Geometry check sheet. Reference: the model listing, model coordinates, mm. Face numbers are marked on the shaded views. A direction names the side the tool comes from. Coordinates: 2 decimals unless noted, no trailing zeros. Loops run counter-clockwise (first coordinate to the right, second up) from the corner with the lowest first, then second, coordinate; pieces in that order, holes last.
from build123d import *
from build123d.topology import SkipClean

# Parameters (mm, degrees)
BOSS_EXTRUDE1_DEPTH      = 42.5
BOSS_EXTRUDE1_DEPTH_BACK = 15
SKETCH1_W                = 40
SKETCH1_H                = 65
SKETCH3_W                = 22.5
SKETCH3_H                = 50
CUT_EXTRUDE2_DEPTH       = 30
SKETCH4_R                = 4.5
CUT_EXTRUDE3_DEPTH       = 10
SKETCH5_W                = 35
SKETCH5_H                = 25
BOSS_EXTRUDE3_DEPTH      = 15
SKETCH6_R                = 3
CUT_EXTRUDE4_DEPTH       = 30
CUT_EXTRUDE5_DEPTH       = 108.964114408
BOSS_EXTRUDE4_DEPTH      = 10
BOSS_EXTRUDE5_OUTLINE_R  = 3
BOSS_EXTRUDE5_DEPTH      = 50
BOSS_EXTRUDE6_START      = -35
SKETCH11_R               = 3
BOSS_EXTRUDE6_DEPTH      = 35
SKETCH12_W               = 14
SKETCH12_H               = 65
SKETCH12_R               = 3.1
SKETCH12_W_2             = 75
SKETCH12_H_2             = 14
BOSS_EXTRUDE7_DEPTH      = 5
SKETCH13_R               = 1.6
CUT_EXTRUDE6_DEPTH       = 115.988042857
CUT_EXTRUDE7_DEPTH       = 12.25
CUT_EXTRUDE7_DEPTH_BACK  = 12.25
SKETCH14_W               = 43.75
SKETCH14_H               = 50
CUT_EXTRUDE8_DEPTH       = 30
CUT_EXTRUDE9_DEPTH       = 115.988042857


# Read off the part's stored shape, not the designer's step: Boss-Extrude5
with BuildPart() as part:
    # Sketch1 → Boss-Extrude1 (new, two sides: drawn at the far end of the back side and taken through both)
    with BuildSketch(Plane.XY.offset(-BOSS_EXTRUDE1_DEPTH_BACK)):
        with Locations((20, 32.5)):
            Rectangle(SKETCH1_W, SKETCH1_H)
    extrude(amount=BOSS_EXTRUDE1_DEPTH + BOSS_EXTRUDE1_DEPTH_BACK)

    # Sketch3 → Cut-Extrude2 (cut)
    with BuildSketch(Plane(origin=(40, 0, 0), x_dir=(0, 0, -1), z_dir=(1, 0, 0))):
        with Locations((-11.25, 40)):
            Rectangle(SKETCH3_W, SKETCH3_H)
    extrude(amount=-CUT_EXTRUDE2_DEPTH, mode=Mode.SUBTRACT)

    # Sketch4 → Cut-Extrude3 (cut)
    with BuildSketch(Plane(origin=(10, 0, 0), x_dir=(0, 0, -1), z_dir=(1, 0, 0))):
        with Locations((-11.25, 26.5)):
            Circle(SKETCH4_R)
    extrude(amount=-CUT_EXTRUDE3_DEPTH, mode=Mode.SUBTRACT)

    # Sketch5 → Boss-Extrude3 (add)
    with BuildSketch(Plane.XZ):
        with Locations((57.5, 30)):
            Rectangle(SKETCH5_W, SKETCH5_H)
    extrude(amount=-BOSS_EXTRUDE3_DEPTH)

    # Sketch6 → Cut-Extrude4 (cut)
    with BuildSketch(Plane.XZ):
        with Locations(Location((32, 29.5, 0), (0, 0, 270))):
            Circle(SKETCH6_R)
        with Locations(Location((64, 29.5, 0), (0, 0, 270))):
            Circle(SKETCH6_R)
    extrude(amount=-CUT_EXTRUDE4_DEPTH, mode=Mode.SUBTRACT)

    # Sketch8 → Cut-Extrude5 (cut, through all)
    with BuildSketch(Plane.XZ):
        Polygon((48.25, 17.5), (42.75, 17.5), (42.75, 23), (53.75, 23), (53.75, 17.5), align=None)
    extrude(amount=-CUT_EXTRUDE5_DEPTH, mode=Mode.SUBTRACT)

    # Sketch9 → Boss-Extrude4 (add)
    with BuildSketch(Plane.XY.offset(42.5)):
        Polygon((0, 65), (0, 0), (75, 0), (75, 15), (40, 15), (40, 65), align=None)
    extrude(amount=BOSS_EXTRUDE4_DEPTH)

    # Boss-Extrude5 outline → Boss-Extrude5 (add)
    with SkipClean():  # the faces are left unmerged after this step: merging them gives an invalid solid
        with BuildSketch(Plane(origin=(0, 15, 0), x_dir=(1, 0, 0), z_dir=(0, 1, 0))):
            Polygon((75, -52.5), (75, -22.5), (53.75, -22.5), (53.75, -23), (42.75, -23), (42.75, -22.5), (40, -22.5), (40, -52.5), align=None)
            with Locations((64, -29.5)):
                Circle(BOSS_EXTRUDE5_OUTLINE_R, mode=Mode.SUBTRACT)
        extrude(amount=BOSS_EXTRUDE5_DEPTH)

    # Sketch11 → Boss-Extrude6 (add)
    with SkipClean():  # the faces are left unmerged after this step: merging them gives an invalid solid
        with BuildSketch(Plane(origin=(0, 65, 0), x_dir=(1, 0, 0), z_dir=(0, 1, 0)).offset(BOSS_EXTRUDE6_START)):
            with Locations(Location((64, -29.5, 0), (0, 0, 90))):
                Circle(SKETCH11_R)
        extrude(amount=BOSS_EXTRUDE6_DEPTH)

    # Sketch12 → Boss-Extrude7 (add)
    # profile 1 of 2: a face of its own
    with SkipClean():  # the faces are left unmerged after this step: merging them gives an invalid solid
        with BuildSketch(Plane.XY.offset(52.5)):
            with Locations((82, 32.5)):
                Rectangle(SKETCH12_W, SKETCH12_H)
            with Locations((82, 53)):
                Circle(SKETCH12_R, mode=Mode.SUBTRACT)
            with Locations((82, 12)):
                Circle(SKETCH12_R, mode=Mode.SUBTRACT)
        # profile 2 of 2: a face of its own
        with BuildSketch(Plane.XY.offset(52.5)):
            with Locations((37.5, -7)):
                Rectangle(SKETCH12_W_2, SKETCH12_H_2)
            with Locations((12, -7)):
                Circle(SKETCH12_R, mode=Mode.SUBTRACT)
            with Locations((63, -7)):
                Circle(SKETCH12_R, mode=Mode.SUBTRACT)
        extrude(amount=-BOSS_EXTRUDE7_DEPTH)

    # Sketch13 → Cut-Extrude6 (cut, through all)
    with SkipClean():  # the faces are left unmerged after this step: merging them gives an invalid solid
        with BuildSketch(Plane(origin=(10, 0, 0), x_dir=(0, 0, -1), z_dir=(1, 0, 0))):
            with Locations((-2.5, 47)):
                Circle(SKETCH13_R)
            with Locations((-20, 47)):
                Circle(SKETCH13_R)
        extrude(amount=-CUT_EXTRUDE6_DEPTH, mode=Mode.SUBTRACT)

    # Sketch14 → Cut-Extrude7 (cut, two sides: drawn at the far end of the back side and taken through both)
    with SkipClean():  # the faces are left unmerged after this step: merging them gives an invalid solid
        with BuildSketch(Plane(origin=(0, 0, 11.25), x_dir=(-1, 0, 0), z_dir=(0, 0, -1)).offset(-CUT_EXTRUDE7_DEPTH_BACK)):
            with Locations((-31.875, 40)):
                Rectangle(SKETCH14_W, SKETCH14_H)
        extrude(amount=CUT_EXTRUDE7_DEPTH + CUT_EXTRUDE7_DEPTH_BACK, mode=Mode.SUBTRACT)

    # Sketch15 → Cut-Extrude8 (cut)
    with SkipClean():  # the faces are left unmerged after this step: merging them gives an invalid solid
        with BuildSketch(Plane(origin=(40, 0, 0), x_dir=(0, 0, -1), z_dir=(1, 0, 0))):
            Polygon((-11.25, 15), (-8.25, 15), (-8.25, 9), (-14.25, 9), (-14.25, 15), align=None)
        extrude(amount=-CUT_EXTRUDE8_DEPTH, mode=Mode.SUBTRACT)

    # Sketch16 → Cut-Extrude9 (cut, through all)
    with SkipClean():  # the faces are left unmerged after this step: merging them gives an invalid solid
        with BuildSketch(Plane(origin=(10, 0, 0), x_dir=(0, 0, -1), z_dir=(1, 0, 0))):
            Polygon((-11.25, 65), (-8.25, 65), (-8.25, 50), (-14.25, 50), (-14.25, 65), align=None)
        extrude(amount=-CUT_EXTRUDE9_DEPTH, mode=Mode.SUBTRACT)


solid = part.part
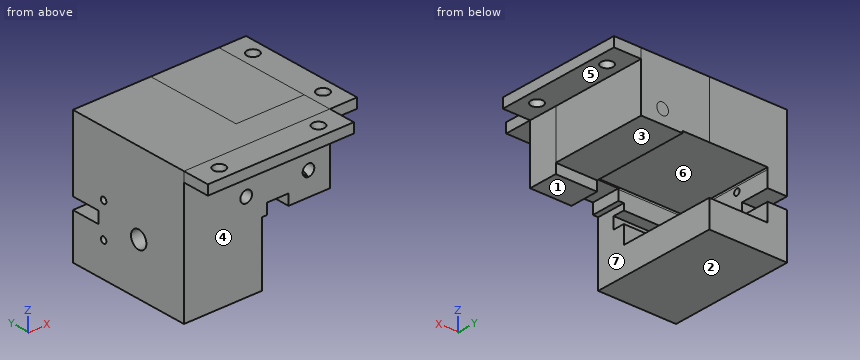
(1) Access from +Z, -Z, +X, -X, +Y, -Y to the whole of each face (thin tool, end or side, straight path). Record for the marked faces 1, 2, 3 and 4.
Findings:
face 1: -Z, +X, +Y, -Y
face 2: -Z, +X, -X, +Y, -Y
face 3: -Z, +X, +Y
face 4: -Z, +X, -X, -Y
(2) Sectioned sample at C-C on x = 12. Record the cut outline in (y, z), and give its area (3 significant figures).
Findings:
outline: (-14, 47.5) - (-10.1, 47.5) - (-10.1, 52.5) - (-14, 52.5) - close; (-3.9, 47.5) - (0, 47.5) - (0, -15) - (65, -15) - (65, -1) - (15, -1) - (15, 8.25) - (9, 8.25) - (9, 14.25) - (15, 14.25) - (15, 23.5) - (65, 23.5) - (65, 52.5) - (-3.9, 52.5) - close
area: 3,170 mm2
(3) Sectioned sample at D-D on z = 20. Record the cut outline in (x, y).
Findings:
outline: (0, 0) - (42.75, 0) - (42.75, 15) - (10, 15) - (10, 45.4) - (0, 45.4) - close; (0, 48.6) - (10, 48.6) - (10, 65) - (0, 65) - close; (53.75, 0) - (75, 0) - (75, 15) - (53.75, 15) - close
(4) Gauge pin test, flat ends, axial feed: pin 1 Ø8 at (x, z) = (34, 16.5) entering from -Y; pin 2 Ø3 at (x, z) = (30, 6.5) entering from +Y; pin 3 Ø12.5 at (y, z) = (48, 38.5) entering from +X; pin 4 Ø11.5 at (y, z) = (26.5, 11.25) entering from -X. Record the tip position at first contact, or that the pin passes through.
Findings:
pin 1: stops at y = 0
pin 2: stops at y = 15
pin 3: stops at x = 75
pin 4: stops at x = 0
(5) Draft check along X on the marked faces 5, 6 and 7. Enter one of: +X half, -X half, draft (parallel to the pull), parting line (faces both ways), or undercut.
Findings:
face 5: draft
face 6: undercut
face 7: +X half
(6) Sectioned sample at B-B on z = 11.25. Record the cut outline in (x, y), and give its area (3 significant figures).
Findings:
outline: (0, 0) - (40, 0) - (40, 9) - (10, 9) - (10, 22) - (0, 22) - close; (0, 31) - (10, 31) - (10, 50) - (0, 50) - close
area: 680 mm2
(7) Sectioned sample at A-A on y = 26.5. Record the cut outline in (x, z).
Findings:
outline: (0, -15) - (40, -15) - (40, -1) - (10, -1) - (10, 6.75) - (0, 6.75) - close; (0, 15.75) - (10, 15.75) - (10, 23.5) - (53.75, 23.5) - (53.75, 22.5) - (75, 22.5) - (75, 47.5) - (89, 47.5) - (89, 52.5) - (0, 52.5) - close; hole circle Ø6 at (32, 29.5); hole circle Ø6 at (64, 29.5)
(8) Scan lines: L1, parallel to Y at x = 82, z = 48; L2, parallel to Y at x = 63, z = 48; L3, parallel to X at y = 11.25, z = 29.5. Record each from-to range of solid material in increasing order.
Findings:
L1: y = 0 to 8.9, 15.1 to 49.9, 56.1 to 65
L2: y = -14 to -10.1, -3.9 to 65
L3: x = 0 to 29, 35 to 61, 67 to 75
